Read the model definition and answer for the solid it produces. Units are mm, in the model's axes. A direction names the side the tool comes from. Coordinates: 2 decimals unless noted, no trailing zeros. Write each loop counter-clockwise with the first axis right and the second up, starting at its lowest first coordinate (ties: lowest second). Pieces come first, ordered by that corner, then holes. Notation, with made-up numbers: (36.25, 9.25) -> (44.25, 9.25) arc R7 cw to (44.25, 17.25) -> close; hole circle Ø8 at (-4, 3). An arc over 180 degrees is marked (long way). Write item = value, one per line. Start each with the question number.
1) For a pull along Y with two mould halves and no side action, classify faces 4 (the face through (2.641, -5, 6)), 5 (the face through (-16.456, 49.477, 21.452)), 6 (the face through (0, 27.744, 6)), 7 (the face through (0, 2, 0)) as released by +Y, released by -Y, zero draft, split by the parting line, or undercut.
2) Section B-B (y = 23) is taken. Determine the outline of the cut face in (x, z), plus the area to 3 significant figures.
3) Section C-C (z = 6.5) is taken. Determine the outline of the cut face in (x, y).
4) Section D-D (z = 16.5) is taken. Determine the outline of the cut face in (x, y).
5) Find the intervals of material crossed by line 1 along X through (y, z) = (22, 23); line 2 along Z through (x, y) = (-3, 12); line 3 along X through (y, z) = (55.5, 20.25), in increasing order. Write a range as from..to.
6) A tool of negligible diameter and unlimited length cuts with its end or side. For faces 1 (the face through (0, -36.372, 6)), 2 (the face through (14.95, 47.08, 22.74)), 3 (the face through (-22.794, -15, 21)), from which of +Z, -Z, +X, -X, +Y, -Y can it reach the whole face along a straight path? Write none if from no direction.
7) Section A-A (z = 23.25) is taken. Determine the outline of the cut face in (x, y), plus the area to 3 significant figures.
8) Flat-ended cylindrical pins translate along their axes: pin 1 Ø4 at (y, z) = (37, 23) entering from +X; pin 2 Ø6 at (x, z) = (-5, 22) entering from +Y; pin 3 Ø2 at (y, z) = (-33.5, 3.5) entering from -X. Find the tip coordinate at first contact, or state that the pin passes through.
from build123d import *

# Parameters (mm, degrees)
F0_W     = 45.5884300172
F0_H     = 84.2695254833
F1_DEPTH = 25.4
F2_T     = -2.54
F3_R     = 17.6135227398
F4_W     = 5.2813845376
F4_H     = 64.1160027434
F5_DEPTH = 7.62
F6_W     = 40.5230503529
F6_H     = 81.5065950155
F7_DEPTH = 2.54


with BuildPart() as f1:
    # F0 (on Top) → F1 (new body)
    with BuildSketch(Plane.XY):
        with BuildLine():
            Line((-22.7942150086, 27.7444738895), (22.7942150086, 27.7444738895))
            ThreePointArc((22.7942150086, 27.7444738895), (16.6249298955, 49.2094594083), (0, 64.1231238842))
            ThreePointArc((0, 64.1231238842), (-16.6249298955, 49.2094594083), (-22.7942150086, 27.7444738895))
        make_face()
        with Locations((0, -14.3902888522)):
            Rectangle(F0_W, F0_H)
    extrude(amount=F1_DEPTH)

    # F2
    f2_openings = [f1.faces().sort_by_distance(p)[0] for p in [
        (0, -1.046307, 25.4),
    ]]
    offset(amount=F2_T, openings=f2_openings)

    # F3
    f3_edges = [f1.edges().sort_by_distance(p)[0] for p in [
        (-22.794215, -14.390289, 0),
        (-16.62493, 49.209459, 0),
        (20.254215, -13.120289, 2.54),
        (14.797736, 47.332252, 2.54),
        (-20.254215, -13.120289, 2.54),
        (-14.797736, 47.332252, 2.54),
        (0, -56.525052, 0),
        (0, -53.985052, 2.54),
        (22.794215, -14.390289, 0),
        (16.62493, 49.209459, 0),
    ]]
    fillet(f3_edges, radius=F3_R)

    # F4 (on face) → F5 (join)
    with BuildSketch(Plane.XY.offset(2.54)):
        with Locations((0, -4.3135274822)):
            Rectangle(F4_W, F4_H)
    extrude(amount=F5_DEPTH)

    # F6 (on face) → F7 (join)
    with BuildSketch(Plane.XY.offset(10.16)):
        with BuildLine():
            ThreePointArc((0, 61.1299425364), (-14.9602203886, 47.3308358732), (-20.4917695373, 27.7444757521))
            Line((-20.4917695373, 27.7444757521), (20.0312808156, 27.7444757521))
            ThreePointArc((20.0312808156, 27.7444757521), (14.639260036, 47.2113810244), (0, 61.1299425364))
        make_face()
        with Locations((-0.2302443609, -13.0088217556)):
            Rectangle(F6_W, F6_H)
    extrude(amount=F7_DEPTH)


solid = f1.part
Answer key:
q1.face_4 = undercut
q1.face_5 = released by +Y
q1.face_6 = undercut
q1.face_7 = zero draft
q2.outline = (-22.79, 17.61) arc R17.61 ccw to (-5.18, 0) -> (5.18, 0) arc R17.61 ccw to (22.79, 17.61) -> (22.79, 25.4) -> (20.25, 25.4) -> (20.25, 20.15) arc R17.61 cw to (18.6, 12.7) -> (-18.6, 12.7) arc R17.61 cw to (-20.25, 20.15) -> (-20.25, 25.4) -> (-22.79, 25.4) -> close; hole (-17.14, 10.16) arc R17.61 ccw to (-2.64, 2.54) -> (-2.64, 10.16) -> close; hole (2.64, 2.54) arc R17.61 ccw to (17.14, 10.16) -> (2.64, 10.16) -> close
q2.area = 363 mm^2
q3.outline = (-18.85, -52.58) -> (18.85, -52.58) -> (18.85, 27.74) arc R36.48 ccw to (0, 59.68) arc R36.48 ccw to (-18.85, 27.74) -> close; (-2.64, -36.37) -> (2.64, -36.37) -> (2.64, 27.74) -> (-2.64, 27.74) -> close; hole (-13.77, -47.5) -> (13.77, -47.5) -> (13.77, 27.74) arc R31.4 ccw to (0, 53.73) arc R31.4 ccw to (-13.77, 27.74) -> close
q4.outline = (-22.76, -56.49) -> (22.76, -56.49) -> (22.76, 27.74) arc R40.39 ccw to (0, 64.08) arc R40.39 ccw to (-22.76, 27.74) -> close; hole (-19.87, -53.6) -> (19.87, -53.6) -> (19.87, 27.74) arc R37.5 ccw to (0, 60.84) arc R37.5 ccw to (-19.87, 27.74) -> close
q5.line_1 = -22.79..-20.25, 20.25..22.79
q5.line_2 = 0..2.54, 10.16..12.7
q5.line_3 = -11.76..-8.16, 8.16..11.76
q6.face_1 = none
q6.face_2 = +Z
q6.face_3 = +Z, -Z, -X, +Y, -Y
q7.outline = (-22.79, -56.53) -> (22.79, -56.53) -> (22.79, 27.74) arc R40.43 ccw to (0, 64.12) arc R40.43 ccw to (-22.79, 27.74) -> close; hole (-20.25, -53.99) -> (20.25, -53.99) -> (20.25, 27.74) arc R37.89 ccw to (0, 61.28) arc R37.89 ccw to (-20.25, 27.74) -> close
q7.area = 751 mm^2
q8.pin_1 = 22.14
q8.pin_2 = 63.08
q8.pin_3 = -16.94
